Autodesk Fusion 360 part; units mm, degrees
sketch "Sketch1" plane through (0, 0, 0) normal (0, 0, 1) x (1, 0, 0)
  circle A0 centre (0, 0) radius 10
  circle A1 centre (0, 0) radius 5
  circle A2 centre (0, 0) radius 1.9
  dimension "d1" = 20
  dimension "d2" = 10
  dimension "d3" = 3.8
extrude "Extrude1" add sketch "Sketch1" along normal blind 3 contours A0 | A1 | A2
extrude "Extrude2" add sketch "Sketch1" along normal blind 13 contours A1 | A2
extrude "Extrude3" add sketch "Sketch1" along normal blind 18 contours A2
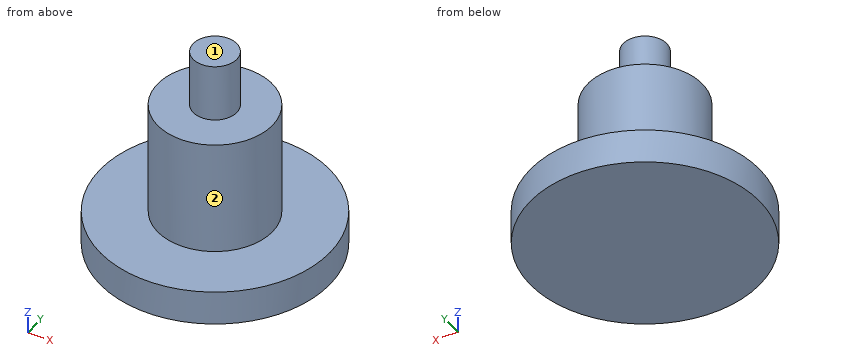
Part model, mm, in its own coordinate system. Face numbers are marked on the shaded views. A direction names the side the tool comes from. Give positions to 0.01 mm unless a question says otherwise; leave off trailing zeros. Order: outer loops, then holes, each group sorted by start corner. A loop starts at its lowest first (then second) coordinate and runs counter-clockwise, first axis right, second up. Notation, with made-up numbers: (-33.75, -11) - (-7.75, -11) arc R23 ccw to (-7.75, 21) - close; hole circle Ø6 at (39.5, -6). An arc over 180 degrees is marked (long way). Use a Markdown table: item, result.
1) Saw through at A-A on y = 0. List the corners of the cut face in (x, z).
Checked values:
| item | result |
|---|---|
| outline | (-10, 0) - (10, 0) - (10, 3) - (5, 3) - (5, 13) - (1.9, 13) - (1.9, 18) - (-1.9, 18) - (-1.9, 13) - (-5, 13) - (-5, 3) - (-10, 3) - close |
2) Saw through at C-C on z = 2. List the corners of the cut face in (x, y), plus the area to 3 significant figures.
Checked values:
| item | result |
|---|---|
| outline | circle Ø20 at (0, 0) |
| area | 314 mm² |
3) Flat gauge pins, fed straight in: P1, Ø4, axis at y = 3.5, z = 6.5, coming from the +X side; P2, Ø10, axis at x = -5.5, z = 9.5, coming from the -Y side; P3, Ø6, axis at x = 6, z = 13, coming from the +Y side; P4, Ø5, axis at x = -7.5, z = 14.5, coming from the -Y side. Where does each tip first touch, or does it go through?
Checked values:
| item | result |
|---|---|
| P1 | x = 4.77 |
| P2 | y = -4.97 |
| P3 | y = 4 |
| P4 | through |
4) 3-axis set-ups, long thin cutter, end or side, ignore diameter. For the marked faces 1 and 2: which of +Z, -Z, +X, -X, +Y, -Y reach the whole face in a straight line?
Checked values:
| item | result |
|---|---|
| face 1 | +Z, +X, -X, +Y, -Y |
| face 2 | +Z |
5) Saw through at D-D on x = -3.75. List the corners of the cut face in (y, z), plus the area to 3 significant figures.
Checked values:
| item | result |
|---|---|
| outline | (-9.27, 0) - (9.27, 0) - (9.27, 3) - (3.31, 3) - (3.31, 13) - (-3.31, 13) - (-3.31, 3) - (-9.27, 3) - close |
| area | 122 mm² |
6) Probe L1, parallel to Z at x = 3.5, y = -7.75; L2, parallel to X at y = 0.25, z = 5.5; L3, parallel to Z at x = 3.75, y = 0.75. List the from-to ranges inside material, lowest first. Write a range as from..to.
Checked values:
| item | result |
|---|---|
| L1 | 0..3 |
| L2 | -4.99..4.99 |
| L3 | 0..13 |
